Autodesk Inventor part; units mm, degrees
ref_plane "YZ Plane" through (0, 0, 0) normal (1, 0, 0) x (0, 1, 0)
ref_plane "XZ Plane" through (0, 0, 0) normal (0, 1, 0) x (-1, 0, 0)
ref_plane "XY Plane" through (0, 0, 0) normal (0, 0, 1) x (1, 0, 0)
sketch "Sketch1" plane through (0, 0, 0) normal (0, 1, 0) x (-1, 0, 0)
  line L0 (-30, 38.5) -> (30, 38.5)
  line L1 (30, 38.5) -> (30, -38.5)
  line L2 (30, -38.5) -> (-30, -38.5)
  line L3 (-30, -38.5) -> (-30, 38.5)
  line L4 (-30, 38.5) -> (30, -38.5) construction
  line L5 (30, 38.5) -> (-30, -38.5) construction
  point P0 (0, 0)
  dimension "d0" = 60
  dimension "d1" = 77
extrude "Extrusion1" add sketch "Sketch1" along normal blind 10
sketch "Sketch2" plane through (0, 10, 0) normal (0, 1, 0) x (1, 0, 0)
  line L0 (27, -35.5) -> (-27, -35.5)
  line L1 (-27, -35.5) -> (-27, 35.5)
  line L2 (-27, 35.5) -> (27, 35.5)
  line L3 (27, 35.5) -> (27, -35.5)
  line L4 (27, -35.5) -> (-27, 35.5) construction
  line L5 (-27, -35.5) -> (27, 35.5) construction
  point P0 (0, 0)
  dimension "d4" = 54
  dimension "d5" = 71
extrude "Extrusion2" cut sketch "Sketch2" against normal blind 8
sketch "Sketch3" plane through (0, 2, 0) normal (0, 1, 0) x (1, 0, 0)
  line L0 (21, -29.5) -> (-21, -29.5)
  line L1 (-21, -29.5) -> (-21, 29.5)
  line L2 (-21, 29.5) -> (21, 29.5)
  line L3 (21, 29.5) -> (21, -29.5)
  line L4 (21, -29.5) -> (-21, 29.5) construction
  line L5 (-21, -29.5) -> (21, 29.5) construction
  point P0 (0, 0)
  dimension "d8" = 42
  dimension "d9" = 59
extrude "Extrusion3" cut sketch "Sketch3" against normal blind 7
fillet "Fillet1" radius 4 4 edges at (-30, 5, 38.5) (30, 5, 38.5) (-30, 5, -38.5) (30, 5, -38.5)
sketch "Sketch4" plane through (0, 0, 0) normal (0, -1, 0) x (1, 0, 0)
  point P0 (0, 0)
sketch "Sketch5" plane through (0, 0, 0) normal (0, -1, 0) x (1, 0, 0)
  point P0 (0, 0)
  point P1 (22.809, 31.309)
  point P2 (22.809, -31.309)
  point P3 (-23, 31.5)
  point P4 (-23, -31.5)
hole "Hole1" at (22.809, 0, 31.309) at (22.809, 0, -31.309) at (-23, 0, -31.5) at (-23, 0, 31.5) direction (0, 1, 0) diameter 2.459 depth 8.8 tip angle 118 countersink diameter 4 countersink angle 90
sketch "Sketch7" plane through (30, 0, 34.5) normal (1, 0, 0) x (0, 0, -1)
  point P0 (34.5, 0)
  point P1 (34.5, 7.5)
hole "Hole2" at (30, 7.5, 0) direction (-1, 0, 0) diameter 6 depth 8.8 tip angle 118
fillet "Fillet2" radius 4 2 edges at (28.5, 10, -1.6583) (28.5, 10, 1.6583)
fillet "Fillet3" radius 2 1 edges at (-21, 1, -29.5)
fillet "Fillet4" radius 2 1 edges at (-21, 1, 29.5)
fillet "Fillet5" radius 2 1 edges at (21, 1, 29.5)
fillet "Fillet6" radius 2 1 edges at (21, 1, -29.5)
equation "\"x\" = 54"
equation "\"z\" = 71"
equation "\"hole\" = 4"
properties part number "cardboardmountfront_sjc"
The model under review builds one solid part; all positions refer to its coordinate system, in mm. A direction names the side the tool comes from. Round coordinates to 2 decimals unless told otherwise and drop trailing zeros. Write each loop counter-clockwise with the first axis right and the second up, starting at its lowest first coordinate (ties: lowest second). Pieces come first, ordered by that corner, then holes. Notation, with made-up numbers: M 42,-16 L 100,-16 A13 ccw 100,-11 Z; hole C 41.5,-34.75 d8. An arc over 180 degrees is marked long. Answer as CSV lines item,"result". Start each with the question number.
Q1. Consider section A-A, the plane y = 3.25. Give the boundary of the cut face in (x, z).
Q2. The part is to be moulded in two halves that separate along Z. For faces 6 (the face through (28.797, 5.07, 37.359)), 7 (the face through (21, 1, 0)), 8 (the face through (28.859, 5.07, -37.297)), say which applies: +Z half, -Z half, draft (parallel to the pull), parting line (faces both ways), or undercut.
Q3. Consider section B-B, the plane z = 0. Give the boundary of the cut face in (x, y), then the cut area to 3 significant figures.
Q4. Clearance check with flat-ended pins moving along their axes: P1, Ø1, axis at x = -21.5, z = 8, coming from the +Y side; P2, Ø4, axis at x = 20, z = -24.5, coming from the -Y side. State where each tip first meets the part, or that it passes through.
Q5. Wall thickness on line 1 along X through (y, z) = (1.7, 31.5); line 2 along X through (y, z) = (4.75, -2); line 3 along Z through (x, y) = (-23, 1.35): over which ranges is each line inside the solid? List them lowest first.
Q6. Tool access review of faces 1 (the face through (-20.4, 0.99, 28.93)), 2 (the face through (27, 0, 1)), 3 (the face through (28.48, 9.14, 4.36)), 4 (the face through (0, 6, 35.5)), 5 (the face through (-28.797, 5.07, -37.359)): name each direction out of +Z, -Z, +X, -X, +Y, -Y from which nothing blocks a thin tool from reaching the whole face with its end or side.
Q7. Consider section C-C, the plane x = -17.5. Give the boundary of the cut face in (y, z).
Q8. Consider section D-D, the plane z = -31.5. State how many separate pieces and enclosed holes the cut face has, then the cut area to 3 significant figures.
Result set:
1,outline,"M -30,-34.5 A4 ccw -26,-38.5 L 26,-38.5 A4 ccw 30,-34.5 L 30,34.5 A4 ccw 26,38.5 L -26,38.5 A4 ccw -30,34.5 Z; hole M -27,-35.5 L 27,-35.5 L 27,35.5 L -27,35.5 Z"
2,face 6,"+Z half"
2,face 7,"undercut"
2,face 8,"-Z half"
3,outline,"M -30,0 L -21,0 L -21,2 L -27,2 L -27,10 L -30,10 Z; M 21,0 L 30,0 L 30,4.5 L 27,4.5 L 27,2 L 21,2 Z"
3,area,"67.5 mm²"
4,P1,"stops at y = 2"
4,P2,"stops at y = 0"
5,line 1,"x = -30 to -24.23, -21.77 to 21.59, 24.02 to 30"
5,line 2,"x = -30 to -27, 27 to 30"
5,line 3,"z = -38.5 to -32.73, -30.27 to 30.27, 32.73 to 38.5"
6,face 1,"+Y, -Y"
6,face 2,"+Z, -Z, +X, -X, -Y"
6,face 3,"+X, +Y"
6,face 4,"+Y"
6,face 5,"-Z, -X, +Y, -Y"
7,outline,"M 0,-38.5 L 10,-38.5 L 10,-35.5 L 2,-35.5 L 2,-29.5 L 0,-29.5 Z; M 0,29.5 L 2,29.5 L 2,35.5 L 10,35.5 L 10,38.5 L 0,38.5 Z"
8,separate pieces,"3"
8,enclosed holes,"0"
8,area,"157 mm²"
